Answer from the drawing. Dimensions are ordinates in mm from the lowest x, y and z of the part. Coordinates: 2 decimals unless noted, no trailing zeros. Loops run counter-clockwise (first coordinate to the right, second up) from the corner with the lowest first, then second, coordinate; pieces in that order, holes last. Notation, with made-up numbers: (70, 74) - (112, 74) arc R21 ccw to (112, 79) - close; hole circle Ø10 at (40, 50.25). An arc over 180 degrees is marked (long way). Write each question's results on one line, items separated by ' | '. Start each with the question number.
1. A cutting plane is placed at A-A on y = 6.75. Determine the outline of the cut face in (x, z).
2. A cutting plane is placed at B-B on x = 43.5. Determine the outline of the cut face in (y, z), then the cut area to 3 significant figures.
3. A cutting plane is placed at C-C on z = 470. Determine the outline of the cut face in (x, y).
4. Find the intervals of material crossed by line 1 along Z through (x, y) = (41, 6.75); line 2 along X through (y, z) = (3.5, 886.5), in increasing order. Write a range as [from, to].
5. Each of these flat-tipped pins is pushed along its axis until it touches: P1, Ø5, axis at y = 7, z = 526.5, coming from the -X side; P2, Ø5, axis at x = 23.5, y = 2.5, coming from the +Z side. Where does it stop, or does it pass through?
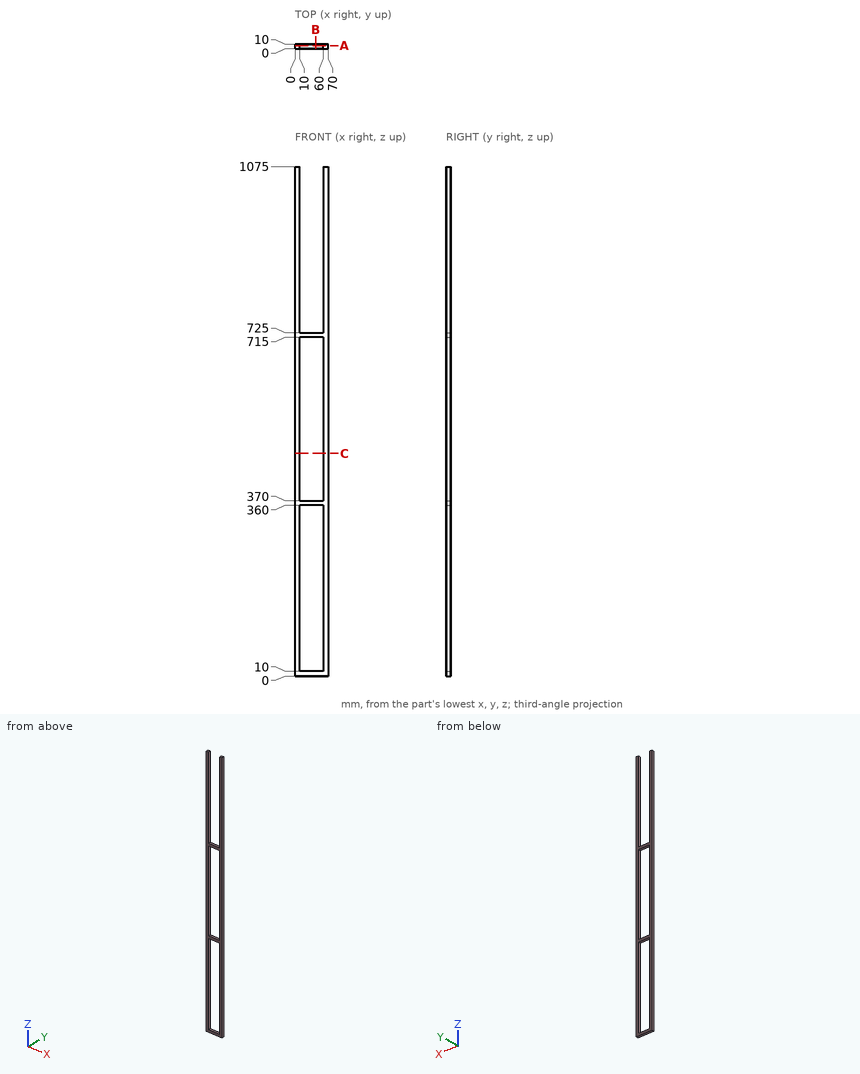
Values:
1) outline: (0, 0) - (70, 0) - (70, 1075) - (60, 1075) - (60, 725) - (10, 725) - (10, 1075) - (0, 1075) - close; hole (10, 10) - (60, 10) - (60, 360) - (10, 360) - close; hole (10, 370) - (60, 370) - (60, 715) - (10, 715) - close
2) outline: (0, 0) - (10, 0) - (10, 10) - (0, 10) - close; (0, 360) - (10, 360) - (10, 370) - (0, 370) - close; (0, 715) - (10, 715) - (10, 725) - (0, 725) - close | area: 300 mm^2
3) outline: (0, 0) - (10, 0) - (10, 10) - (0, 10) - close; (60, 0) - (70, 0) - (70, 10) - (60, 10) - close
4) line 1: [0, 10], [360, 370], [715, 725] | line 2: [0, 10], [60, 70]
5) P1: x = 0 | P2: z = 725
